For this review, take the finished solid that the model builds, in its own axes (mm). Give positions to 0.01 mm unless a question says otherwise; leave off trailing zeros. Write each loop counter-clockwise with the first axis right and the second up, starting at its lowest first coordinate (ties: lowest second). Pieces come first, ordered by that corner, then holes. Notation, with made-up numbers: (60.5, -34.75) -> (108.5, -34.75) arc R22 cw to (108.5, -2.75) -> close; hole circle Ø5 at (47.25, -16.75). An arc over 180 degrees is marked (long way). Write item = value, one per line.
Autodesk Inventor part; units mm, degrees
ref_plane "Work Plane1" through (0, 0, -6.35) normal (0, 0, 1) x (1, 0, 0)
ref_plane "Work Plane2" through (0, 0, -41.875) normal (0, 0, 1) x (1, 0, 0)
ref_plane "Work Plane3" through (0, 0, -35.525) normal (0, 0, 1) x (1, 0, 0)
sketch "Sketch1" plane through (0, 0, 0) normal (0, 0, 1) x (1, 0, 0)
  line L0 (0, 0) -> (114.0582, 0)
  line L1 (114.0582, 0) -> (114.0582, 95.9104)
  line L2 (114.0582, 95.9104) -> (0, 95.9104)
  line L3 (0, 95.9104) -> (0, 0)
  line L4 (59.1, 17.1) -> (59.1, 59.1)
  line L5 (59.1, 59.1) -> (17.1, 59.1)
  line L6 (17.1, 59.1) -> (17.1, 17.1)
  line L7 (17.1, 17.1) -> (59.1, 17.1)
  line L8 (59.1, 17.1) -> (17.1, 59.1) construction
  line L9 (59.1, 59.1) -> (17.1, 17.1) construction
  circle A0 centre (38.1, 38.1) radius 38.1 construction
  circle A1 centre (38.1, 38.1) radius 20.2
  line L10 (45.4323, 38.1) -> (41.7662, 31.75)
  line L11 (41.7662, 31.75) -> (34.4338, 31.75)
  line L12 (34.4338, 31.75) -> (30.7677, 38.1)
  line L13 (30.7677, 38.1) -> (34.4338, 44.45)
  line L14 (34.4338, 44.45) -> (41.7662, 44.45)
  line L15 (41.7662, 44.45) -> (45.4323, 38.1)
  circle A2 centre (38.1, 38.1) radius 21.59 construction
  line L16 (38.1, 38.1) -> (81.0382, 62.8904) construction
  circle A3 centre (81.0382, 62.8904) radius 27.94 construction
  circle A4 centre (81.0382, 62.8904) radius 23.8125 construction
  circle A5 centre (81.0382, 62.8904) radius 17.4625
  circle A6 centre (38.1, 38.1) radius 14.2875
  line L17 (85.0105, 18.6054) -> (38.1, 38.1) construction
  circle A7 centre (81.0382, 62.8904) radius 33.02 construction
  circle A8 centre (38.1, 38.1) radius 25.4 construction
  circle A9 centre (38.1, 38.1) radius 11.1125
  line L18 (81.0382, 62.8904) -> (81.0382, 42.1545)
  circle A10 centre (81.0382, 42.1545) radius 2.0828 construction
  circle A11 centre (39.5622, 74.901) radius 10.16
  circle A12 centre (39.5622, 74.901) radius 6.35
  circle A13 centre (81.0382, 42.1545) radius 6.35 construction
  circle A14 centre (38.1, 38.1) radius 26.67 construction
  line L19 (85.0105, 18.6054) -> (87.4474, 24.4692)
  line L20 (85.0105, 18.6054) -> (82.5737, 12.7416)
  line L21 (87.4474, 24.4692) -> (77.6267, 28.5504)
  line L22 (82.5737, 12.7416) -> (72.2567, 17.029)
  circle A15 centre (103.8982, 10.16) radius 10.16
  circle A16 centre (103.8982, 10.16) radius 6.35
  circle A17 centre (10.16, 10.16) radius 10.16
  circle A18 centre (38.1, 38.1) radius 32.258 construction
  circle A19 centre (10.16, 10.16) radius 6.35
  point P0 (20.1395, 56.0605)
  point P1 (56.0605, 20.1395)
  point P2 (81.0382, 44.2373)
  point P3 (81.0382, 45.4279)
  point P4 (98.9961, 73.2584)
  point P5 (63.0804, 73.2584)
  point P6 (81.0382, 48.5045)
  point P7 (79.1467, 21.0422)
  dimension "d10" = 34.925
  dimension "d17" = 4.1656
  dimension "d25" = 12.7
  dimension "d0" = 42
  dimension "d1" = 42
  dimension "d2" = 76.2
  dimension "d3" = 40.4
  dimension "d4" = 12.7
  dimension "d5" = 43.18
  dimension "d6" = 55.88
  dimension "d7" = 49.5808
  dimension "d8" = 47.625
  dimension "d11" = 28.575
  dimension "d13" = 30
  dimension "d14" = 5.08
  dimension "d15" = 50.8
  dimension "d16" = 22.225
  dimension "d18" = 1.1906
  dimension "d21" = 360
  dimension "d23" = 20.32
  dimension "d24" = 12.7
  dimension "d26" = 3.0766
  dimension "d30" = 5.08
  dimension "d33" = 50.8
  dimension "d34" = 6.35
  dimension "d35" = 6.35
  dimension "d36" = 20.32
  dimension "d37" = 64.516
  dimension "d38" = 12.7
ref_plane "Work Plane1" through (0, 0, -6.35) normal (0, 0, 1) x (1, 0, 0)
ref_plane "Work Plane2" through (0, 0, -41.875) normal (0, 0, 1) x (1, 0, 0)
ref_plane "Work Plane3" through (0, 0, -35.525) normal (0, 0, 1) x (1, 0, 0)
ref_plane "Work Plane4" through (0, 0, -92.675) normal (0, 0, 1) x (1, 0, 0)
ref_plane "Work Plane5" through (0, 0, -99.025) normal (0, 0, 1) x (1, 0, 0)
sketch "Sketch2" plane through (0, 0, -6.35) normal (0, 0, 1) x (1, 0, 0)
  line L0 (114.0582, 95.9104) -> (0, 95.9104)
  line L1 (0, 95.9104) -> (0, 0)
  line L2 (0, 0) -> (114.0582, 0)
  line L3 (114.0582, 0) -> (114.0582, 95.9104)
  circle A0 centre (81.0382, 62.8904) radius 17.4625
  circle A1 centre (38.1, 38.1) radius 11.1125
sketch "Sketch3" plane through (0, 0, -41.875) normal (0, 0, 1) x (1, 0, 0)
  line L0 (114.0582, 95.9104) -> (0, 95.9104)
  line L1 (114.0582, 0) -> (114.0582, 95.9104)
  circle A0 centre (81.0382, 62.8904) radius 17.4625
  line L2 (0, 0) -> (114.0582, 0)
  line L3 (0, 95.9104) -> (0, 0)
  circle A1 centre (38.1, 38.1) radius 14.2875
sketch "Sketch4" plane through (0, 0, -35.525) normal (0, 0, 1) x (1, 0, 0)
  line L0 (114.0582, 95.9104) -> (0, 95.9104)
  line L1 (0, 95.9104) -> (0, 0)
  line L2 (0, 0) -> (114.0582, 0)
  line L3 (114.0582, 0) -> (114.0582, 95.9104)
  circle A0 centre (81.0382, 62.8904) radius 17.4625
  circle A1 centre (38.1, 38.1) radius 14.2875
sketch "Sketch5" plane through (0, 0, -92.675) normal (0, 0, 1) x (1, 0, 0)
  line L0 (0, 95.9104) -> (0, 0)
  line L1 (114.0582, 95.9104) -> (0, 95.9104)
  line L2 (0, 0) -> (114.0582, 0)
  line L3 (114.0582, 0) -> (114.0582, 95.9104)
  circle A0 centre (81.0382, 62.8904) radius 17.4625
sketch "Sketch6" plane through (0, 0, -99.025) normal (0, 0, 1) x (1, 0, 0)
  line L0 (0, 95.9104) -> (0, 0)
  line L1 (0, 0) -> (114.0582, 0)
  line L2 (114.0582, 0) -> (114.0582, 95.9104)
  line L3 (114.0582, 95.9104) -> (0, 95.9104)
  circle A0 centre (81.0382, 62.8904) radius 17.4625
extrude "Extrusion1" add sketch "Sketch1" along normal blind 6.35 contours L3 A17 L0 | A17 L7 L4 L5 L6 L3 L2 L1 A15 L0 | A17 L6 L7 | A15 L1 L0 | A15 | A17 L7 L6 | L6 L5 L4 L7 A17 | A1 | A6 | A11 | A12 | A16 | A19
hole "Hole1" at (39.5622, 74.901, 0) at (10.16, 10.16, 0) at (103.8982, 10.16, 0) direction (0, 0, 1) diameter 4.9784 end through all
hole "Hole2" at (81.0382, 42.1545, 0) at (98.9961, 73.2584, 0) at (63.0804, 73.2584, 0) direction (0, 0, 1) diameter 3.9624 end through all
hole "Hole3" at (79.1467, 21.0422, 0) direction (0, 0, 1) diameter 6.5278 end through all
hole "Hole4" at (20.1395, 56.0605, 0) at (56.0605, 20.1395, 0) direction (0, 0, 1) diameter 4.9784 end through all countersink diameter 10.795 countersink angle 82
equation "\"d30\" = d14"
properties part number "Main Outline"
(1) The part is to be moulded in two halves that separate along Y. For faces 1 (the face through (58.709, 19.792, 3.136)), 2 (the face through (56, 0, 3)), 3 (the face through (58, 95.91, 3)), 4 (the face through (114.058, 47, 3)), say which applies: released by +Y, released by -Y, zero draft, split by the parting line, or undercut.
Answers below:
face_1 = undercut
face_2 = released by -Y
face_3 = released by +Y
face_4 = zero draft
(2) Take a section at A-A (y = 38.1). Write out the cut boundary in (x, z).
Answers below:
outline = (0, 0) -> (26.99, 0) -> (26.99, 6.35) -> (0, 6.35) -> close; (49.21, 0) -> (114.06, 0) -> (114.06, 6.35) -> (49.21, 6.35) -> close
(3) To check wall thickness, follow probe 1 along X at (y, z) = (10.16, 4); probe 2 along X at (y, z) = (21.5, 4.25) (3 decimals); probe 3 along X at (y, z) = (75, 5). State the ranges of each line that lie inside material, in increasing order.
Answers below:
probe_1 = 0 to 7.67, 12.65 to 101.41, 106.39 to 114.06
probe_2 = 0 to 53.976, 58.145 to 75.915, 82.378 to 114.058
probe_3 = 0 to 37.07, 42.05 to 62.14, 64.02 to 68.46, 93.62 to 98.05, 99.94 to 114.06
(4) Take a section at D-D (z = 4.75). Count the separate pieces of the cut face and the enclosed holes in it, plus the area to 3 significant figures.
Answers below:
separate_pieces = 1
enclosed_holes = 11
area = 9,430 mm^2
(5) Take a section at C-C (x = 10.16). Write out the cut boundary in (y, z), plus the area to 3 significant figures.
Answers below:
outline = (0, 0) -> (7.67, 0) -> (7.67, 6.35) -> (0, 6.35) -> close; (12.65, 0) -> (95.91, 0) -> (95.91, 6.35) -> (12.65, 6.35) -> close
area = 577 mm^2
(6) Take a section at B-B (y = 10.16). Write out the cut boundary in (x, z), plus the area to 3 significant figures.
Answers below:
outline = (0, 0) -> (7.67, 0) -> (7.67, 6.35) -> (0, 6.35) -> close; (12.65, 0) -> (101.41, 0) -> (101.41, 6.35) -> (12.65, 6.35) -> close; (106.39, 0) -> (114.06, 0) -> (114.06, 6.35) -> (106.39, 6.35) -> close
area = 661 mm^2
(7) For pin 1 (4 mm diameter, centred on x = 10.16, y = 10.16, fed in from +Z), flat-tipped, find the tip position at first contact; note if it passes through.
Answers below:
pin_1 = through
